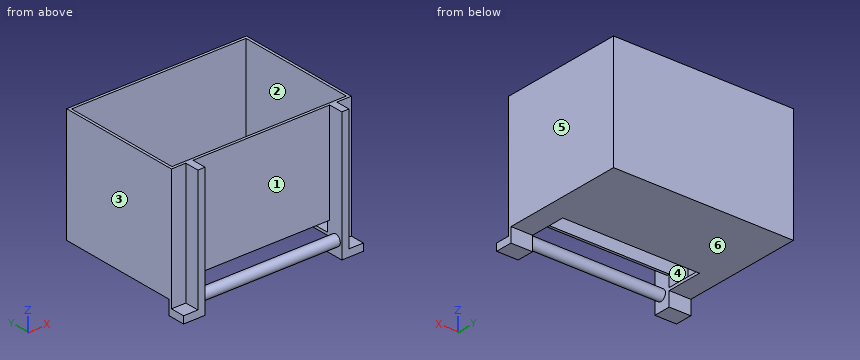
from build123d import *

# Parameters (mm, degrees)
F0_W      = 25.4
F0_H      = 50.8
F1_DEPTH  = 457.2
F2_W      = 50.8
F2_H      = 25.4
F3_DEPTH  = 50.8
F4_R      = 19.05
F5_DEPTH  = 241.3
F7_W      = 50.8
F7_H      = 431.8
F8_DEPTH  = 9.525
F11_DEPTH = 9.525
F12_W     = 9.525
F12_H     = 406.4
F13_DEPTH = 431.8
F14_W     = 615.95
F14_H     = 9.525
F15_DEPTH = 396.875


# Not quite as in the source:
# - a feature names something its author has since deleted; it is built from what else it names


with BuildPart() as f1:
    # F0 (on Top) → F1 (new body)
    with BuildSketch(Plane.XY):
        with Locations((-254, 0)):
            Rectangle(F0_W, F0_H)
    extrude(amount=F1_DEPTH)

    # F2 (on face) → F3 (join)
    with BuildSketch(Plane(origin=(-266.7, 0, 0), x_dir=(0, -1, 0), z_dir=(-1, 0, 0))):
        with Locations((0, 12.7)):
            Rectangle(F2_W, F2_H)
    extrude(amount=F3_DEPTH)

    # F4 (on face) → F5 (join)
    with BuildSketch(Plane.YZ.offset(-241.3)):
        with Locations((0, 50.8)):
            Circle(F4_R)
    extrude(amount=F5_DEPTH)

    # F6: F1 across plane


with BuildPart() as f1_1:
    add(f1.part)
    add(f1.part.mirror(Plane.YZ))

    # F7 (on face) → F8 (join)
    with BuildSketch(Plane(origin=(0, 25.4, 0), x_dir=(-1, 0, 0), z_dir=(0, 1, 0))):
        Polygon((241.3, 0), (317.5, 0), (317.5, 25.4), (266.7, 25.4), (266.7, 457.2), (241.3, 457.2), (241.3, 101.6), align=None)
        with Locations((292.1, 241.3)):
            Rectangle(F7_W, F7_H)
        Polygon((0, 101.6), (241.3, 101.6), (241.3, 457.2), (0, 457.2), (-241.3, 457.2), (-241.3, 101.6), align=None)
        Polygon((-241.3, 0), (-241.3, 101.6), (-241.3, 457.2), (-317.5, 457.2), (-317.5, 0), align=None)
    extrude(amount=F8_DEPTH)

    # F10 (on offset) → F11 (join)
    with BuildSketch(Plane.XY.offset(50.8)):
        Polygon((-307.975, 34.925), (-241.3, 34.925), (-241.3, 161.925), (241.3, 161.925), (241.3, 34.925), (307.975, 34.925), (307.975, 466.725), (-307.975, 466.725), align=None)
    extrude(amount=F11_DEPTH)

    # F12 (on face) → F13 (join)
    with BuildSketch(Plane(origin=(0, 34.925, 0), x_dir=(-1, 0, 0), z_dir=(0, 1, 0))):
        with Locations((-312.7375, 254)):
            Rectangle(F12_W, F12_H)
        with Locations((312.7375, 254)):
            Rectangle(F12_W, F12_H)
    extrude(amount=F13_DEPTH)

    # F14 (on face) → F15 (join, through all)
    with BuildSketch(Plane.XY.offset(60.325)):
        with Locations((0, 461.9625)):
            Rectangle(F14_W, F14_H)
    extrude(amount=F15_DEPTH)


solid = f1_1.part
Design review of the part built by this model. Coordinates are the model's own, in mm. Face numbers are marked on the shaded views. A direction names the side the tool comes from. Round coordinates to 2 decimals unless told otherwise and drop trailing zeros. Write each loop counter-clockwise with the first axis right and the second up, starting at its lowest first coordinate (ties: lowest second). Pieces come first, ordered by that corner, then holes. Notation, with made-up numbers: (-21, 60.25) -> (29, 60.25) arc R24 cw to (29, 70.25) -> close; hole circle Ø9 at (58.5, 39). An arc over 180 degrees is marked (long way). One line per item, written item: value. Start each with the question number.
Q1. Add section A-A (x = -99). Give the boundary of the cut face in (y, z) (3 decimals), then the cut area to 3 significant figures.
Q2. Tool access review of the marked faces 1, 2 and 3: name each direction out of +Z, -Z, +X, -X, +Y, -Y from which nothing blocks a thin tool from reaching the whole face with its end or side.
Q3. Add section C-C (z = 258). Give the boundary of the cut face in (x, y) (3 decimals).
Q4. Add section B-B (y = 292). Give the boundary of the cut face in (x, z) (3 decimals).
Q5. To check wall thickness, follow probe 1 along Y at (x, z) = (-242.5, 79) (3 decimals); probe 2 along Y at (x, z) = (-96.5, 309) (3 decimals); probe 3 along X at (y, z) = (144.5, 324) (3 decimals). State the ranges of each line that lie inside material, in increasing order.
Q6. The part is to be moulded in two halves that separate along X. For the marked faces 4, 5 and 6, say which applies: pulls with the +X half, pulls with the -X half, needs draft (parallel to the pull), parting line crosses it, or undercut.
Q7. Add section D-D (y = 0). Give the boundary of the cut face in (x, z).
Q8. Insertion check: P1, Ø10.5, axis at x = 29.5, z = 54.5, coming from the -Y side; P2, Ø15, axis at y = 5.5, z = 216.5, coming from the +X side; P3, Ø2, axis at x = 106, y = 282, coming from the +Z side (3 decimals). Each pin has a flat end and moves straight along its axis. Give the tip position at first contact, or say it passes through.
Response:
1. outline: circle Ø38.1 at (0, 50.8); (25.4, 101.6) -> (34.925, 101.6) -> (34.925, 457.2) -> (25.4, 457.2) -> close; (161.925, 50.8) -> (466.725, 50.8) -> (466.725, 457.2) -> (457.2, 457.2) -> (457.2, 60.325) -> (161.925, 60.325) -> close
1. area: 11,200 mm^2
2. face 1: +Z, -Z, -Y
2. face 2: +Z
2. face 3: +Z, -Z, -X, +Y, -Y
3. outline: (-317.5, 25.4) -> (-266.7, 25.4) -> (-266.7, -25.4) -> (-241.3, -25.4) -> (-241.3, 25.4) -> (241.3, 25.4) -> (241.3, -25.4) -> (266.7, -25.4) -> (266.7, 25.4) -> (317.5, 25.4) -> (317.5, 466.725) -> (-317.5, 466.725) -> close; hole (-307.975, 34.925) -> (307.975, 34.925) -> (307.975, 457.2) -> (-307.975, 457.2) -> close
4. outline: (-317.5, 50.8) -> (317.5, 50.8) -> (317.5, 457.2) -> (307.975, 457.2) -> (307.975, 60.325) -> (-307.975, 60.325) -> (-307.975, 457.2) -> (-317.5, 457.2) -> close
5. probe 1: y = -25.4 to 34.925, 457.2 to 466.725
5. probe 2: y = 25.4 to 34.925, 457.2 to 466.725
5. probe 3: x = -317.5 to -307.975, 307.975 to 317.5
6. face 4: undercut
6. face 5: pulls with the +X half
6. face 6: needs draft
7. outline: (-317.5, 0) -> (-241.3, 0) -> (-241.3, 31.75) -> (241.3, 31.75) -> (241.3, 0) -> (317.5, 0) -> (317.5, 25.4) -> (266.7, 25.4) -> (266.7, 457.2) -> (241.3, 457.2) -> (241.3, 69.85) -> (-241.3, 69.85) -> (-241.3, 457.2) -> (-266.7, 457.2) -> (-266.7, 25.4) -> (-317.5, 25.4) -> close
8. P1: stops at y = -19.05
8. P2: stops at x = 266.7
8. P3: stops at z = 60.325
